Verification items for the finished model (mm, model axes). Round coordinates to 2 decimals unless told otherwise and drop trailing zeros. Write each loop counter-clockwise with the first axis right and the second up, starting at its lowest first coordinate (ties: lowest second). Pieces come first, ordered by that corner, then holes. Notation, with made-up numbers: M 64.25,-40 L 109.25,-40 A17 ccw 109.25,-20 Z; hole C 60.25,35 d3. An arc over 180 degrees is marked long. One line per item, written item: value. Start each with the question number.
Item 1: Thickness scan on probe 1 along Y at (x, z) = (-43.5, 0.6); probe 2 along X at (y, z) = (2, 0.4); probe 3 along X at (y, z) = (4.5, 0.25). Record the ranges inside material, lowest first. Write a range as from..to.
Item 2: Section check D-D, the plane x = -25. Record the cut outline in (y, z), then the cut area to 3 significant figures.
Item 3: Section check C-C, the plane x = 25. Record the cut outline in (y, z), then the cut area to 3 significant figures.
Item 4: Section check A-A, the plane y = 0. Record the cut outline in (x, z), then the cut area to 3 significant figures.
Item 5: Draft check along X on faces 1 (the face through (-29.76, -3.65, 0.41)), 2 (the face through (-48.289, -20.696, 0.406)), 3 (the face through (42.579, 16.845, 0.406)), 4 (the face through (48.289, 20.696, 0.406)). Enter one of: +X half, -X half, draft (parallel to the pull), parting line (faces both ways), or undercut.
Item 6: Section check B-B, the plane z = 0.35. Record the cut outline in (x, y), then the cut area to 3 significant figures.
Autodesk Inventor part; units mm, degrees
ref_plane "YZ Plane" through (0, 0, 0) normal (1, 0, 0) x (0, 1, 0)
ref_plane "XZ Plane" through (0, 0, 0) normal (0, 1, 0) x (-1, 0, 0)
ref_plane "XY Plane" through (0, 0, 0) normal (0, 0, 1) x (1, 0, 0)
sketch "Skizze2" plane through (0, 0, 0) normal (0, 0, 1) x (1, 0, 0)
  line L0 (-50, -22.5) -> (50, -22.5)
  line L1 (50, -22.5) -> (50, 22.5)
  line L2 (50, 22.5) -> (-50, 22.5)
  line L3 (-50, 22.5) -> (-50, -22.5)
  line L4 (-50, -22.5) -> (50, 22.5) construction
  line L5 (50, -22.5) -> (-50, 22.5) construction
  point P0 (0, 0)
  dimension "d0" = 100
  dimension "d1" = 45
extrude "Extrusion1" add sketch "Skizze2" along normal blind 0.8
fillet "Rundung1" radius 6 4 edges at (-50, 22.5, 0.4) (50, 22.5, 0.4) (50, -22.5, 0.4) (-50, -22.5, 0.4)
sketch "Skizze3" plane through (0, 0, 0.8) normal (0, 0, 1) x (1, 0, 0)
  line L0 (-50, 22.5) -> (50, 22.5) construction
  line L1 (50, 22.5) -> (50, -22.6939) construction
  line L2 (50, -22.6939) -> (-50, -22.6939) construction
  line L3 (-50, -22.6939) -> (-50, 22.5) construction
  line L4 (-50, 16.5) -> (-50, -16.5)
  line L5 (44, 22.5) -> (-44, 22.5)
  point P0 (0, 0)
  dimension "d6" = 100
decal "Aufkleber1"
sketch "Skizze4" plane through (0, 0, 0.8) normal (0, 0, 1) x (1, 0, 0)
  circle A0 centre (-25, 0) radius 6
  line L0 (44, 22.5) -> (-44, 22.5)
  line L1 (-50, 16.5) -> (-50, -16.5)
  circle A1 centre (25, 0) radius 3.5
  line L2 (50, -16.5) -> (50, 16.5)
  point P0 (0, 0)
  dimension "d10" = 22.5
  dimension "d11" = 25
  dimension "d12" = 12
  dimension "d15" = 25
  dimension "d16" = 7
extrude "Extrusion2" cut sketch "Skizze4" against normal through all
sketch "Skizze5" plane through (0, 0, 0.8) normal (0, 0, 1) x (1, 0, 0)
  circle A0 centre (-43.5, 16) radius 1.25
  circle A1 centre (43.5, 16) radius 1.25
  circle A2 centre (43.5, -16) radius 1.25
  circle A3 centre (-43.5, -16) radius 1.25
  line L0 (0, 31.5) -> (0, -31.5) construction
  line L1 (-71.1379, 0) -> (70.1897, 0) construction
  line L2 (44, 22.5) -> (-44, 22.5) construction
  line L3 (-50, 16.5) -> (-50, -16.5) construction
  point P0 (0, 0)
  dimension "d17" = 2.5
  dimension "d18" = 6.5
  dimension "d19" = 6.5
extrude "Extrusion3" cut sketch "Skizze5" against normal through all
properties part number "EW_MessingplatteBedienelemente" material "Messing"
Response values:
1. probe 1: y = -22.5..-17.25, -14.75..14.75, 17.25..22.5
1. probe 2: x = -50..-30.66, -19.34..22.13, 27.87..50
1. probe 3: x = -50..-28.97, -21.03..50
2. outline: M -22.5,0 L -6,0 L -6,0.8 L -22.5,0.8 Z; M 6,0 L 22.5,0 L 22.5,0.8 L 6,0.8 Z
2. area: 26.4 mm2
3. outline: M -22.5,0 L -3.5,0 L -3.5,0.8 L -22.5,0.8 Z; M 3.5,0 L 22.5,0 L 22.5,0.8 L 3.5,0.8 Z
3. area: 30.4 mm2
4. outline: M -50,0 L -31,0 L -31,0.8 L -50,0.8 Z; M -19,0 L 21.5,0 L 21.5,0.8 L -19,0.8 Z; M 28.5,0 L 50,0 L 50,0.8 L 28.5,0.8 Z
4. area: 64.8 mm2
5. face 1: undercut
5. face 2: -X half
5. face 3: undercut
5. face 4: +X half
6. outline: M -50,-16.5 A6 ccw -44,-22.5 L 44,-22.5 A6 ccw 50,-16.5 L 50,16.5 A6 ccw 44,22.5 L -44,22.5 A6 ccw -50,16.5 Z; hole C -43.5,-16 d2.5; hole C -43.5,16 d2.5; hole C -25,0 d12; hole C 25,0 d7; hole C 43.5,-16 d2.5; hole C 43.5,16 d2.5
6. area: 4,300 mm2
